Work out the finished part from the listing and answer in its coordinate system (mm). Face numbers are marked on the shaded views. A direction names the side the tool comes from. Give positions to 0.01 mm unless a question says otherwise; leave off trailing zeros. Loops run counter-clockwise (first coordinate to the right, second up) from the corner with the lowest first, then second, coordinate; pieces in that order, holes last. Notation, with made-up numbers: (-16.75, -10.75) - (-1.75, -10.75) arc R30 cw to (-1.75, 12.25) - close; hole circle Ø2 at (14, -32.5). An arc over 180 degrees is marked (long way). One line per item, written item: value.
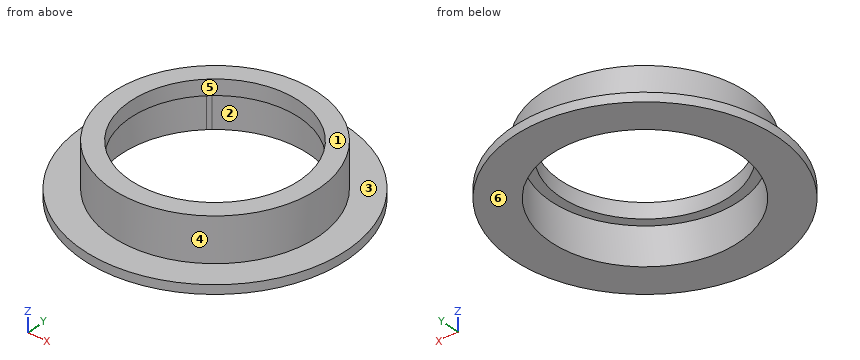
Autodesk Inventor part; units mm, degrees
ref_plane "YZ Plane" through (0, 0, 0) normal (1, 0, 0) x (0, 1, 0)
ref_plane "XZ Plane" through (0, 0, 0) normal (0, 1, 0) x (-1, 0, 0)
ref_plane "XY Plane" through (0, 0, 0) normal (0, 0, 1) x (1, 0, 0)
sketch "Sketch1" plane through (0, 0, 0) normal (0, 0, 1) x (1, 0, 0)
  circle A0 centre (0, 0) radius 9.4
  circle A1 centre (0, 0) radius 10.45
  circle A2 centre (0, 0) radius 7
  line L0 (0, 0) -> (0, 1.4)
  line L1 (0, 1.4) -> (-5.6, 1.4)
  line L2 (-6, 1.8) -> (-6, 5.8)
  line L3 (-5.6, 6.2) -> (0, 6.2)
  arc A3 (-6, 1.8) -> (-5.6, 1.4) centre (-5.6, 1.8) ccw
  arc A4 (-5.6, 6.2) -> (-6, 5.8) centre (-5.6, 5.8) ccw
  line L4 (0, 1.4) -> (5.6, 1.4)
  line L5 (6, 1.8) -> (6, 5.8)
  line L6 (5.6, 6.2) -> (0, 6.2)
  arc A5 (5.6, 1.4) -> (6, 1.8) centre (5.6, 1.8) ccw
  arc A6 (6, 5.8) -> (5.6, 6.2) centre (5.6, 5.8) ccw
  circle A7 centre (0, -9.4) radius 1.05
  line L7 (5.8828, 6.0828) -> (6.2306, 7.0384)
  line L8 (5.8828, 6.0828) -> (6.8997, 6.0828) construction
  circle A8 centre (6.2306, 7.0384) radius 1.0741
  circle A9 centre (-6.2306, 7.0384) radius 1.0741
  line L9 (0, 6.2) -> (0, 1.4)
  line L10 (-4.5, 2.55) -> (4.5, 2.55)
  line L11 (4.5, 2.55) -> (4.5, 5.05)
  line L12 (4.5, 5.05) -> (-4.5, 5.05)
  line L13 (-4.5, 5.05) -> (-4.5, 2.55)
  line L14 (-4.5, 2.55) -> (4.5, 5.05) construction
  line L15 (4.5, 2.55) -> (-4.5, 5.05) construction
  line L16 (-10.45, 0) -> (-11.45, 0)
  circle A10 centre (0, 0) radius 11.45
  line L17 (-11.45, 0) -> (-14.65, 0)
  circle A11 centre (0, 0) radius 14.65
  point P0 (-6, 1.4)
  point P1 (-6, 6.2)
  point P2 (1.0484, -9.3414)
  point P3 (-1.0484, -9.3414)
  point P4 (7.1035, 7.6644)
  point P5 (6.7461, 7.9808)
  point P6 (5.387, 7.7033)
  point P7 (6.9929, 6.2816)
  point P8 (-7.1035, 7.6644)
  point P9 (-6.9929, 6.2816)
  point P10 (-5.387, 7.7033)
  point P11 (-6.7461, 7.9808)
  point P12 (0, 3.8)
  dimension "d1" = 20.9
  dimension "d0" = 18.8
  dimension "d8" = 14
  dimension "d18" = 1.4
  dimension "d19" = 6
  dimension "d20" = 4.8
  dimension "d21" = 0.4
  dimension "d22" = 70
  dimension "d25" = 9
  dimension "d26" = 2.5
  dimension "d31" = 1
  dimension "d32" = 3.2
extrude "Extrusion7" add sketch "Sketch1" along normal blind 1.7 contours A0 A8 A1 A7 | A0 A8 A1 | A7 A0 | A7 A1 A9 A0 | A0 A9 A1 A8 | A10 | A1 A8 | A9 A1 A0 | A9 A1 picked at (0, -9.7457)
extrude "Extrusion8" add sketch "Sketch1" against normal blind 3.2 from surface at 0 contours A10
extrude "Extrusion9" add sketch "Sketch1" against normal blind 1 from surface at -3.2 contours A10 | A11
properties part number "fingerprint sensor seal"
1. Section C-C (z = -1.8) is taken. Write down the section's boundary in (x, y).
Output:
outline: circle Ø22.9 at (0, 0); hole (-7.1, 7.66) arc R10.45 ccw (long way) to (7.1, 7.66) arc R1.07 ccw to (6.75, 7.98) arc R10.45 ccw to (-6.75, 7.98) arc R1.07 ccw to start
2. Section B-B (y = 2.5) is taken. Write down the section's boundary in (x, z), and give its area (3 significant figures).
Output:
outline: (-14.44, -4.2) - (-10.15, -4.2) - (-10.15, 0) - (-9.06, 0) - (-9.06, 1.7) - (-11.17, 1.7) - (-11.17, -3.2) - (-14.44, -3.2) - close; (9.06, 0) - (10.15, 0) - (10.15, -4.2) - (14.44, -4.2) - (14.44, -3.2) - (11.17, -3.2) - (11.17, 1.7) - (9.06, 1.7) - close
area: 22.3 mm²
3. Find the intervals of material crossed by line 1 along Y through (x, z) = (0, 1.45); line 2 along Y through (x, z) = (0, -2.9); line 3 along Z through (x, y) = (13.5, -4.75), in increasing order.
Output:
line 1: y = -11.45 to -9.4, 9.4 to 11.45
line 2: y = -11.45 to -10.45, 10.45 to 11.45
line 3: z = -4.2 to -3.2
4. The mould has two halves that part along X. Classify the marked faces 4, 5 and 6: released by +X, released by -X, zero draft, split by the parting line, or undercut.
Output:
face 4: split by the parting line
face 5: undercut
face 6: zero draft
5. Section D-D (z = 0.45) is taken. Write down the section's boundary in (x, y), and give its area (3 significant figures).
Output:
outline: circle Ø22.9 at (0, 0); hole circle Ø18.8 at (0, 0)
area: 134 mm²
6. Flat-ended cylindrical pins translate along their axes: pin 1 Ø1.5 at (x, z) = (5, -3) entering from -Y; pin 2 Ø3 at (y, z) = (4, 0.5) entering from -X. Find the tip coordinate at first contact, or state that the pin passes through.
Output:
pin 1: stops at y = -14.01
pin 2: stops at x = -11.17
7. Section A-A (x = 0) is taken. Write down the section's boundary in (y, z).
Output:
outline: (-14.65, -4.2) - (-10.45, -4.2) - (-10.45, 0) - (-9.4, 0) - (-9.4, 1.7) - (-11.45, 1.7) - (-11.45, -3.2) - (-14.65, -3.2) - close; (9.4, 0) - (10.45, 0) - (10.45, -4.2) - (14.65, -4.2) - (14.65, -3.2) - (11.45, -3.2) - (11.45, 1.7) - (9.4, 1.7) - close
8. For the marked faces 1, 2 and 3, determine the directions among +Z, -Z, +X, -X, +Y, -Y from which every point of the face is accessible in a straight line to the end or side of a thin tool.
Output:
face 1: +Z, +X, -X, +Y, -Y
face 2: -Z
face 3: +Z
